Work out the finished part from the listing and answer in its coordinate system (mm). Coordinates: 2 decimals unless noted, no trailing zeros. Loops run counter-clockwise (first coordinate to the right, second up) from the corner with the lowest first, then second, coordinate; pieces in that order, holes last. Notation, with made-up numbers: (-39.75, -21.75) - (-1.75, -21.75) arc R26 ccw to (-1.75, 0.25) - close; hole circle Ø8 at (88, -33.75). An arc over 180 degrees is marked (long way). Write each question's results on one line, items separated by ' | '. Start each with the question number.
1. A cutting plane is placed at D-D on z = 10. Determine the outline of the cut face in (x, y) (3 decimals), then the cut area to 3 significant figures.
2. Determine the mould class of faces 1 (the cylindrical face through (-50.676, 1.565, 12.555)), 2 (the cylindrical face through (-63.02, 1.61, 0.45)), 3 (the flat face through (0, 2, 13)) for opening direction X: released by +X, released by -X, zero draft, split by the parting line, or undercut.
3. A cutting plane is placed at A-A on z = 12.7. Determine the outline of the cut face in (x, y) (3 decimals).
4. Find the intervals of material crossed by line 1 along Z through (x, y) = (-9.5, 1.6); line 2 along X through (y, z) = (0.9, 15); line 3 along Z through (x, y) = (-7, 1.85), in increasing order. Write a range as [from, to].
5. A cutting plane is placed at C-C on y = 1.05. Determine the outline of the cut face in (x, z) (1 decimal), then the cut area to 3 significant figures.
6. A cutting plane is placed at B-B on x = -8.5. Determine the outline of the cut face in (y, z) (3 decimals), then the cut area to 3 significant figures.
Autodesk Inventor part; units mm, degrees
ref_plane "YZ Plane" through (0, 0, 0) normal (1, 0, 0) x (0, 1, 0)
ref_plane "XZ Plane" through (0, 0, 0) normal (0, 1, 0) x (-1, 0, 0)
ref_plane "XY Plane" through (0, 0, 0) normal (0, 0, 1) x (1, 0, 0)
sketch "Sketch1" plane through (0, 0, 0) normal (0, 1, 0) x (-1, 0, 0)
  line L0 (0, 0) -> (63.5, 0)
  line L1 (63.5, 0) -> (63.5, 25.4)
  line L2 (63.5, 25.4) -> (0, 25.4)
  line L3 (0, 25.4) -> (0, 0)
  circle A0 centre (9.525, 12.7) radius 3.302
  circle A1 centre (53.975, 12.7) radius 3.302
  line L4 (9.525, 12.7) -> (53.975, 12.7) construction
  line L5 (31.75, 25.4) -> (31.75, 0) construction
  point P0 (31.75, 12.7)
  dimension "d0" = 63.5
  dimension "d2" = 25.4
  dimension "d3" = 44.45
  dimension "d4" = 6.604
extrude "Extrusion1" add sketch "Sketch1" along normal blind 3.175
fillet "Fillet1" radius 1.5875 4 edges at (0, 1.5875, 25.4) (0, 1.5875, 0) (-63.5, 1.5875, 0) (-63.5, 1.5875, 25.4)
properties part number "Wheel Mount Support Plate" material "Aluminum 6061"
Values:
1) outline: (-63.5, 0) - (-55.876, 0) - (-55.876, 3.175) - (-63.5, 3.175) - close; (-52.074, 0) - (-11.426, 0) - (-11.426, 3.175) - (-52.074, 3.175) - close; (-7.624, 0) - (0, 0) - (0, 3.175) - (-7.624, 3.175) - close | area: 177 mm^2
2) face 1: undercut | face 2: released by -X | face 3: released by +X
3) outline: (-63.5, 0) - (-57.277, 0) - (-57.277, 3.175) - (-63.5, 3.175) - close; (-50.673, 0) - (-12.827, 0) - (-12.827, 3.175) - (-50.673, 3.175) - close; (-6.223, 0) - (0, 0) - (0, 3.175) - (-6.223, 3.175) - close
4) line 1: [0, 9.4], [16, 25.4] | line 2: [-63.5, -56.34], [-51.61, -11.89], [-7.16, 0] | line 3: [0, 10.57], [14.83, 25.4]
5) outline: (-63.5, 1.6) arc R1.6 ccw to (-61.9, 0) - (-1.6, 0) arc R1.6 ccw to (0, 1.6) - (0, 23.8) arc R1.6 ccw to (-1.6, 25.4) - (-61.9, 25.4) arc R1.6 ccw to (-63.5, 23.8) - close; hole circle Ø6.6 at (-54, 12.7); hole circle Ø6.6 at (-9.5, 12.7) | area: 1,540 mm^2
6) outline: (0, 0) - (3.175, 0) - (3.175, 9.561) - (0, 9.561) - close; (0, 15.839) - (3.175, 15.839) - (3.175, 25.4) - (0, 25.4) - close | area: 60.7 mm^2
